```python
from build123d import *

# Parameters (mm, degrees)
SKETCH_W    = 254
SKETCH_H    = 304.8
SKETCH_R    = 3.175
PAD_DEPTH   = 12.999999
FILLET_R    = 2.54
FILLET001_R = 2.54
FILLET002_R = 2.54


with BuildPart() as part:
    # Sketch → Pad (new body)
    with BuildSketch(Plane.XY):
        with Locations((127, 152.4)):
            Rectangle(SKETCH_W, SKETCH_H)
        with Locations((9.525, 25.4)):
            Circle(SKETCH_R, mode=Mode.SUBTRACT)
        with Locations((9.525, 101.6)):
            Circle(SKETCH_R, mode=Mode.SUBTRACT)
        with Locations((9.525, 254)):
            Circle(SKETCH_R, mode=Mode.SUBTRACT)
        with Locations((244.475, 254)):
            Circle(SKETCH_R, mode=Mode.SUBTRACT)
        with Locations((244.475, 101.6)):
            Circle(SKETCH_R, mode=Mode.SUBTRACT)
        with Locations((244.475, 25.4)):
            Circle(SKETCH_R, mode=Mode.SUBTRACT)
    extrude(amount=PAD_DEPTH)

    # Fillet
    fillet_edges = [part.edges().sort_by_distance(p)[0] for p in [
        (0, 0, 6.5),
    ]]
    fillet(fillet_edges, radius=FILLET_R)

    # Fillet001
    fillet001_edges = [part.edges().sort_by_distance(p)[0] for p in [
        (254, 0, 6.5),
    ]]
    fillet(fillet001_edges, radius=FILLET001_R)

    # Fillet002
    fillet002_edges = [part.edges().sort_by_distance(p)[0] for p in [
        (0, 304.8, 6.5),
        (254, 304.8, 6.5),
    ]]
    fillet(fillet002_edges, radius=FILLET002_R)


solid = part.part
```
Work out the finished part from the listing and answer in its coordinate system (mm). Coordinates: 2 decimals unless noted, no trailing zeros. Answer as CSV lines item,"result".
Q1. Find the intervals of material crossed by probe 1 along X at (y, z) = (254, 8), in increasing order.
Findings:
probe 1,"x = 0 to 6.35, 12.7 to 241.3, 247.65 to 254"
Q2. This flat-tipped pin is pushed along its axis until it touches: pin 1 (5.5 mm diameter, centred on x = 244.475, y = 254, fed in from +Z). Where does it stop, or does it pass through?
Findings:
pin 1,"passes through"
Q3. For a pull along Y with two mould halves and no side action, classify faces 1 (the face through (125, 0, 6)), 2 (the face through (241.3, 101.7, 6.4)), 3 (the face through (125, 155, 0)) as +Y half, -Y half, draft (parallel to the pull), parting line (faces both ways), or undercut.
Findings:
face 1,"-Y half"
face 2,"undercut"
face 3,"draft"
